Could you check a few things on this drawing? It's one solid part, dimensions in mm from its lowest x, y, z. A direction names the side the tool comes from. Coordinates: 2 decimals unless noted, no trailing zeros. Loops run counter-clockwise (first coordinate to the right, second up) from the corner with the lowest first, then second, coordinate; pieces in that order, holes last.
1) Thinking about a two-plate mould opening in Z: for the marked faces 1, 2 and 3, which applies, released by +Z, released by -Z, zero draft, split by the parting line, or undercut?
2) Imagine slicing it at B-B on x = 33. Please give me the cut outline in (y, z) (1 decimal).
3) Imagine slicing it at D-D on y = 72. Please give me the cut outline in (x, z) (1 decimal).
4) If I drill on line 1 along Y through (x, z) = (51.5, 22.5); line 2 along Z through (x, y) = (31.5, 38.5); line 3 along X through (y, z) = (16, 23) (1 decimal), over which ranges is the centre line in solid material (lowest first)?
5) Imagine slicing it at C-C on x = 42.5. Please give me the cut outline in (y, z).
6) For the marked faces 4 and 5, which set-ups out of +Z, -Z, +X, -X, +Y, -Y let a thin tool reach every point of the face, with its end or its side?
7) Imagine slicing it at A-A on z = 20.5. Please give me the cut outline in (x, y), plus the area to 3 significant figures.
8) Will these pins go through, and if not, where does the flat tip stop? P1, Ø4, axis at x = 16.5, z = 30.5, coming from the +Y side; P2, Ø5, axis at y = 56.5, z = 26.5, coming from the +X side (1 decimal).
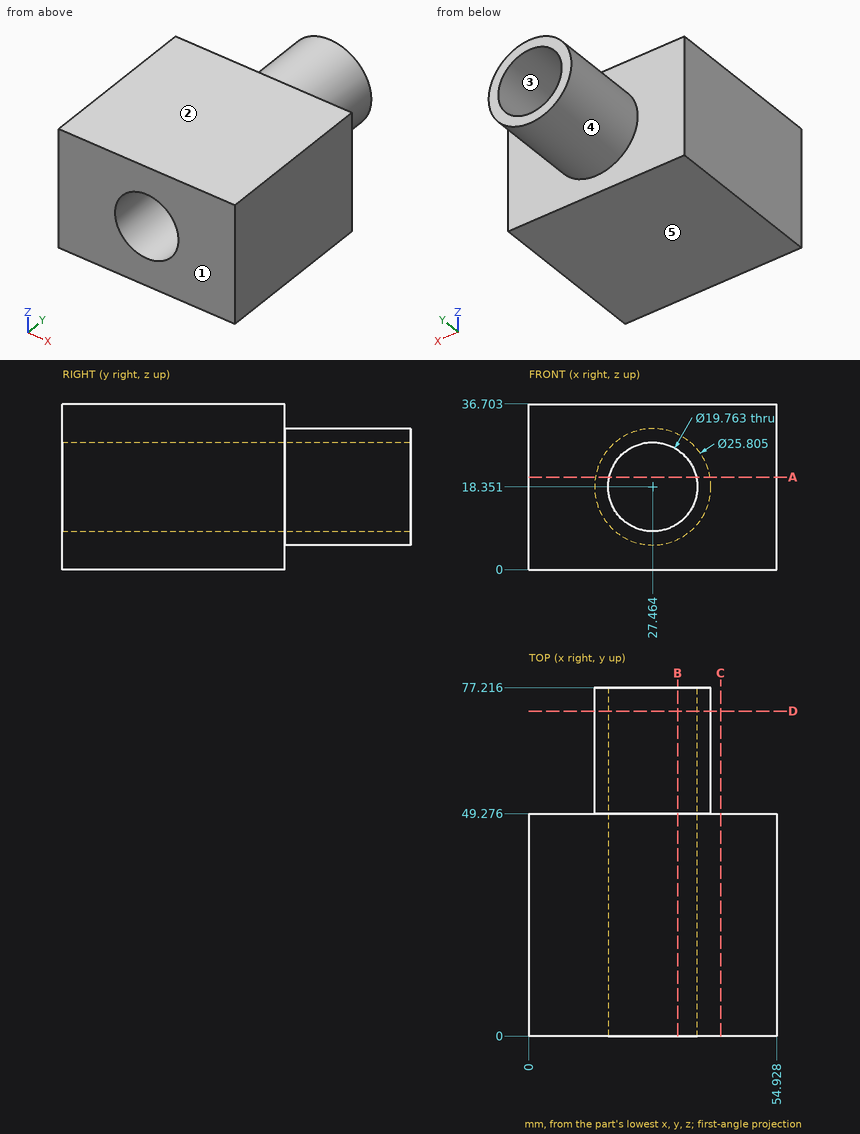
Filled in:
1. face 1: zero draft
1. face 2: released by +Z
1. face 3: undercut
2. outline: (0, 0) - (49.3, 0) - (49.3, 6.7) - (77.2, 6.7) - (77.2, 10.2) - (0, 10.2) - close; (0, 26.5) - (77.2, 26.5) - (77.2, 30) - (49.3, 30) - (49.3, 36.7) - (0, 36.7) - close
3. outline: circle Ø25.8 at (27.5, 18.4); hole circle Ø19.8 at (27.5, 18.4)
4. line 1: y = 0 to 49.28
4. line 2: z = 0 to 9.33, 27.37 to 36.7
4. line 3: x = 0 to 18.7, 36.2 to 54.9
5. outline: (0, 0) - (49.28, 0) - (49.28, 36.7) - (0, 36.7) - close
6. face 4: +Y
6. face 5: -Z, +X, -X, +Y, -Y
7. outline: (0, 0) - (17.82, 0) - (17.82, 77.22) - (14.74, 77.22) - (14.74, 49.28) - (0, 49.28) - close; (37.11, 0) - (54.93, 0) - (54.93, 49.28) - (40.19, 49.28) - (40.19, 77.22) - (37.11, 77.22) - close
7. area: 1,930 mm2
8. P1: stops at y = 49.28
8. P2: stops at x = 39.1
